from build123d import *

# Parameters (mm, degrees)
SKETCH2_R           = 292.1
SKETCH2_R_2         = 152.4
BOSS_EXTRUDE1_DEPTH = 203.2
FILLET1_R           = 101.6
SHELL1_T            = -6.35


with BuildPart() as part:
    # Sketch2 → Boss-Extrude1 (new body)
    with BuildSketch(Plane(origin=(0, 0, 0), x_dir=(0, 0, -1), z_dir=(1, 0, 0))):
        Circle(SKETCH2_R)
        Circle(SKETCH2_R_2, mode=Mode.SUBTRACT)
    extrude(amount=-BOSS_EXTRUDE1_DEPTH)

    # Fillet1
    fillet1_edges = [part.edges().sort_by_distance(p)[0] for p in [
        (0, 0, 292.1),
        (-203.2, 0, 292.1),
    ]]
    fillet(fillet1_edges, radius=FILLET1_R - 0.0001)  # a hair under: the kernel refuses the full size

    # Shell1
    shell1_openings = [part.faces().sort_by_distance(p)[0] for p in [
        (-101.6, 0, 152.4),
    ]]
    offset(amount=SHELL1_T, openings=shell1_openings, kind=Kind.INTERSECTION)


solid = part.part
Verification items for the finished model (mm, model axes). A direction names the side the tool comes from. Round coordinates to 2 decimals unless told otherwise and drop trailing zeros. Loops run counter-clockwise (first coordinate to the right, second up) from the corner with the lowest first, then second, coordinate; pieces in that order, holes last. Notation, with made-up numbers: (-5.5, -23) - (37.5, -23) arc R28 cw to (37.5, 1) - close; hole circle Ø1 at (85, 35). An arc over 180 degrees is marked (long way). Answer in a Markdown table with one row per item. Add a question column.
Q1. Gauge pin test, flat ends, axial feed: pin 1 (2 mm diameter, centred on x = -175, z = -119.5, fed in from +Y); pin 2 (1 mm diameter, centred on y = -201.5, z = -76.5, fed in from +X); pin 3 (6 mm diameter, centred on x = -149, y = 192.5, fed in from -Z). Record the tip position at first contact, or that the pin passes through.
Q2. Section check C-C on x = -118. Enter the section's corners in (y, z), plus the area to 3 significant figures.
Q3. Material ranges on line 1 (Y direction, x = -101.55, z = 0); line 2 (X direction, y = -153, z = -87); line 3 (X direction, y = -173.5, z = -90.5), recorded low to high.
Q4. Release check for a two-part mould opening along Z. For faces 1 (the face through (-199.98, -92.73, 120.94)), 2 (the face through (-203.2, 128, 86)) record: pulls with the +Z half, pulls with the -Z half, needs draft (parallel to the pull), parting line crosses it, or undercut.
Q5. Tool access check on faces 3 (the face through (-3.13, -92.73, 120.94)), 4 (the face through (-6.35, 128, 86)). Record the directions out of +Z, -Z, +X, -X, +Y, -Y that give a thin tool (end or side, any length) a straight path to the whole face; none if there is none.
Q6. Section check D-D on x = -185. Enter the section's corners in (y, z), plus the area to 3 significant figures.
Found:
| question | item | result |
|---|---|---|
| 1 | pin 1 | stops at y = 233.02 |
| 1 | pin 2 | stops at x = -3.01 |
| 1 | pin 3 | stops at z = -207.33 |
| 2 | outline | circle Ø581.54 at (0, 0); hole circle Ø568.66 at (0, 0) |
| 2 | area | 11,600 mm² |
| 3 | line 1 | y = -292.1 to -285.75, 285.75 to 292.1 |
| 3 | line 2 | x = -203.2 to -196.85, -6.35 to 0 |
| 3 | line 3 | x = -203.07 to -196.71, -6.49 to -0.13 |
| 4 | face 1 | undercut |
| 4 | face 2 | needs draft |
| 5 | face 3 | +X, -X |
| 5 | face 4 | none |
| 6 | outline | circle Ø497.05 at (0, 0); hole circle Ø473.02 at (0, 0) |
| 6 | area | 18,300 mm² |
